CAD build for the part. Positions are in the model's coordinates, mm. Face numbers are marked on the shaded views. Coordinates: 2 decimals unless noted, no trailing zeros. Order: outer loops, then holes, each group sorted by start corner. A loop starts at its lowest first (then second) coordinate and runs counter-clockwise, first axis right, second up. Notation, with made-up numbers: M 12,6.5 L 39,6.5 A24 ccw 39,35.5 Z; hole C 9.5,37 d7. An arc over 180 degrees is marked long. Write item = value, one per line.
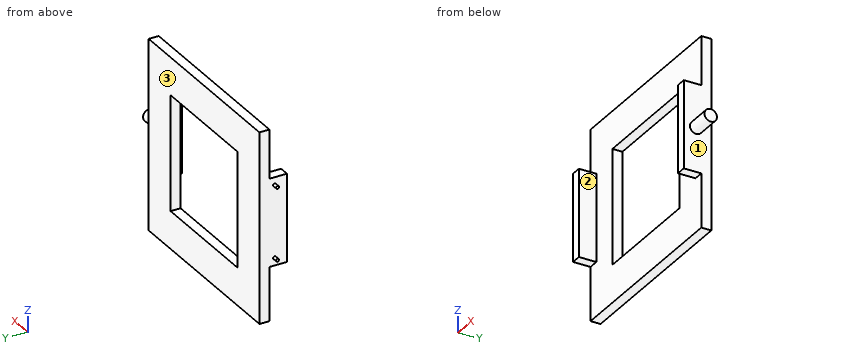
from build123d import *

# Parameters (mm, degrees)
SKETCH1_W             = 76
SKETCH1_H             = 76
SKETCH1_W_2           = 46
SKETCH1_H_2           = 46
BOSS_EXTRUDE2_DEPTH   = 4
SKETCH7_R             = 0.6
BOSS_EXTRUDE5_DEPTH   = 2
BOSS_EXTRUDE5_2_DEPTH = 2
SKETCH8_W             = 35
SKETCH8_H             = 11
BOSS_EXTRUDE6_DEPTH   = 4
SKETCH9_W             = 35
SKETCH9_H             = 11
BOSS_EXTRUDE7_DEPTH   = 4
SKETCH10_R            = 2.5
BOSS_EXTRUDE8_DEPTH   = 10


with BuildPart() as part:
    # Sketch1 → Boss-Extrude2 (new body)
    with BuildSketch(Plane(origin=(0, 0, 0), x_dir=(1, 0, 0), z_dir=(0, 1, 0))):
        with Locations((38, 38)):
            Rectangle(SKETCH1_W, SKETCH1_H)
        with Locations((38, 38)):
            Rectangle(SKETCH1_W_2, SKETCH1_H_2, mode=Mode.SUBTRACT)
    extrude(amount=BOSS_EXTRUDE2_DEPTH)



with BuildPart() as body_2:
    # Sketch7 → Boss-Extrude5 (new body)
    with BuildSketch(Plane.ZY):
        with Locations((-51.45, -2.06)):
            Circle(SKETCH7_R)
    extrude(amount=BOSS_EXTRUDE5_DEPTH)


with BuildPart() as body_3:
    # Sketch7 → Boss-Extrude5 2 (new body)
    with BuildSketch(Plane.ZY):
        with Locations((-22.55, -2.06)):
            Circle(SKETCH7_R)
    extrude(amount=BOSS_EXTRUDE5_2_DEPTH)


with BuildPart() as part_1:
    add(part.part)

    add(body_2.part)  # Boss-Extrude6 merges body 2

    add(body_3.part)  # Boss-Extrude6 merges body 3
    # Sketch8 → Boss-Extrude6 (add)
    with BuildSketch(Plane.ZY):
        with Locations((-37, -1.5)):
            Rectangle(SKETCH8_W, SKETCH8_H)
    extrude(amount=-BOSS_EXTRUDE6_DEPTH)

    # Sketch9 → Boss-Extrude7 (add)
    with BuildSketch(Plane(origin=(76, 0, 0), x_dir=(0, 0, -1), z_dir=(1, 0, 0))):
        with Locations((37, -1.5)):
            Rectangle(SKETCH9_W, SKETCH9_H)
    extrude(amount=-BOSS_EXTRUDE7_DEPTH)

    # Sketch10 → Boss-Extrude8 (add)
    with BuildSketch(Plane(origin=(76, 0, 0), x_dir=(0, 0, -1), z_dir=(1, 0, 0))):
        with Locations((36.93, -2.06)):
            Circle(SKETCH10_R)
    extrude(amount=BOSS_EXTRUDE8_DEPTH)


solid = part_1.part
(1) Slice it at B-B, the plane x = 25. Write the cut outline in (y, z).
Evaluation:
outline = M 0,-76 L 4,-76 L 4,-61 L 0,-61 Z; M 0,-15 L 4,-15 L 4,0 L 0,0 Z
(2) Slice it at D-D, the plane x = 66.5. Write the cut outline in (y, z).
Evaluation:
outline = M 0,-76 L 4,-76 L 4,0 L 0,0 Z
(3) Pull direction X, two halves, no side cores. Call the marked faces 1, 2 and 3: +X half, -X half, draft (parallel to the pull), parting line (faces both ways), or undercut.
Evaluation:
face_1 = +X half
face_2 = undercut
face_3 = draft
(4) Wall check: line 1 (X direction, y = 1.5, z = -49); line 2 (X direction, y = -5.25, z = -50); line 3 (Z direction, x = 16.5, y = 1.5). Give the ranges that are in metal, low to high. Write a range as from..to.
Evaluation:
line_1 = 0..15, 61..76
line_2 = 0..4, 72..76
line_3 = -76..-61, -15..0
(5) Pin check, flat tips, straight feed: pin 1 Ø8 at (x, z) = (20, -55.5) entering from +Y; pin 2 Ø6 at (y, z) = (-1.5, -17.5) entering from +X; pin 3 Ø3.5 at (y, z) = (-4, -38) entering from -X; pin 4 Ø3 at (x, y) = (2.5, -5) entering from +Z. Stop position of each tip, or through.
Evaluation:
pin_1 = through
pin_2 = 76
pin_3 = 0
pin_4 = -19.5
(6) Slice it at A-A, the plane z = -30.5. Write the cut outline in (x, y).
Evaluation:
outline = M 0,-7 L 4,-7 L 4,0 L 15,0 L 15,4 L 0,4 Z; M 61,0 L 72,0 L 72,-7 L 76,-7 L 76,4 L 61,4 Z
(7) Slice it at C-C, the plane z = -62. Write the cut outline in (x, y), then the cut area to 3 significant figures.
Evaluation:
outline = M 0,0 L 76,0 L 76,4 L 0,4 Z
area = 304 mm²
